Solid Edge part; units mm, degrees
sketch "Sketch1" plane through (0, 0, 0) normal (1, 0, 0) x (0, 1, 0)
  line L0 (-8, 8) -> (-8, 3)
  line L1 (-8, 3) -> (-6, 3)
  line L2 (-6, 3) -> (-6, 6)
  line L3 (-6, 6) -> (-2, 6)
  line L4 (-2, 6) -> (-2, -6)
  line L5 (-2, -6) -> (-6, -6)
  line L6 (-6, -6) -> (-6, -3)
  line L7 (-6, -3) -> (-8, -3)
  line L8 (-8, -3) -> (-8, -8)
  line L9 (-8, -8) -> (0, -8)
  line L10 (0, -8) -> (0, 8)
  line L11 (0, 8) -> (-8, 8)
  dimension "D1" = 2
extrude "Protrusion1" add sketch "Sketch1" along normal mid plane 200
fillet "Round_1" radius 0.4 12 edges at (0, -8, 8) (0, 0, 8) (0, -8, 3) (0, -6, 3) (0, -6, 6) (0, -2, 6) (0, -2, -6) (0, -6, -6) (0, -6, -3) (0, -8, -3) (0, -8, -8) (0, 0, -8)
properties material "Stainless steel"
Part model, mm, in its own coordinate system. A direction names the side the tool comes from. Give positions to 0.01 mm unless a question says otherwise; leave off trailing zeros. Write each loop counter-clockwise with the first axis right and the second up, starting at its lowest first coordinate (ties: lowest second). Pieces come first, ordered by that corner, then holes. Notation, with made-up numbers: (-39, 11) -> (-35, 11) arc R6 ccw to (-35, 22) -> close; hole circle Ø7 at (-39.5, -19). An arc over 180 degrees is marked (long way). Put each result on its own line as item: value. Start each with the question number.
Item 1: Cut at B-B (z = 0). List the corners of the cut face in (x, y), then the cut area to 3 significant figures.
Item 2: Pull direction Z, two halves, no side cores. Call faces 3 (the face through (-1, -4, -8)), 4 (the face through (-1, -8, -5)), 5 (the face through (-1, -4, -6)): pulls with the +Z half, pulls with the -Z half, needs draft (parallel to the pull), parting line crosses it, or undercut.
Item 3: Cut at A-A (x = 69.5). List the corners of the cut face in (y, z).
Item 4: Wall check: L1, parallel to Z at x = 86, y = -3; L2, parallel to Z at x = -91.5, y = -7.5; L3, parallel to Y at x = -51, z = 3.5. Give the ranges that are in metal, low to high. Write a range as [from, to].
Item 5: Which spindle directions (+Z, -Z, +X, -X, +Y, -Y) get a long thin tool onto all of the face, cutting with end or side? Do faces 1 (the face through (-1, -2, 0)), 2 (the face through (-1, 0, 0)). Say none if no direction does.
Answer list:
1. outline: (-100, -2) -> (100, -2) -> (100, 0) -> (-100, 0) -> close
1. area: 400 mm2
2. face 3: pulls with the -Z half
2. face 4: needs draft
2. face 5: undercut
3. outline: (-8, -7.6) arc R0.4 ccw to (-7.6, -8) -> (-0.4, -8) arc R0.4 ccw to (0, -7.6) -> (0, 7.6) arc R0.4 ccw to (-0.4, 8) -> (-7.6, 8) arc R0.4 ccw to (-8, 7.6) -> (-8, 3.4) arc R0.4 ccw to (-7.6, 3) -> (-6.4, 3) arc R0.4 ccw to (-6, 3.4) -> (-6, 5.6) arc R0.4 cw to (-5.6, 6) -> (-2.4, 6) arc R0.4 cw to (-2, 5.6) -> (-2, -5.6) arc R0.4 cw to (-2.4, -6) -> (-5.6, -6) arc R0.4 cw to (-6, -5.6) -> (-6, -3.4) arc R0.4 ccw to (-6.4, -3) -> (-7.6, -3) arc R0.4 ccw to (-8, -3.4) -> close
4. L1: z = [-8, -6], [6, 8]
4. L2: z = [-8, -3], [3, 8]
4. L3: y = [-8, -6], [-2, 0]
5. face 1: +X, -X
5. face 2: +Z, -Z, +X, -X, +Y
